The listing builds one solid part. Answer for the finished solid, in the listing's coordinates (mm). A direction names the side the tool comes from. Give positions to 0.01 mm unless a question says otherwise; leave off trailing zeros. Loops run counter-clockwise (first coordinate to the right, second up) from the corner with the lowest first, then second, coordinate; pieces in that order, holes last. Notation, with made-up numbers: (29, 8.5) - (83, 8.5) arc R26 ccw to (83, 36.5) - close; hole circle Ø5 at (-10, 30). An arc over 180 degrees is marked (long way). Write item = value, one per line. Start each with the question number.
1) Flat-ended cylindrical pins translate along their axes: P1, Ø5, axis at y = 4, z = -19.5, coming from the +X side; P2, Ø2, axis at x = -2, y = 5.5, coming from the -Z side; P3, Ø6, axis at y = -5, z = 2, coming from the -X side. Find the tip coordinate at first contact, or state that the pin passes through.
2) Which of the six approach directions +Z, -Z, +X, -X, +Y, -Y give full straight-line access (tool end or side, diameter ignored) to faces 1 (the flat face through (0, 0, 9.525)), 2 (the flat face through (-2, 3, 0))?
3) The part is cut by section D-D on z = 6. Write down the section's boundary in (x, y).
4) Consider probe 1 along Z at (x, y) = (-5.25, 2.5) (3 decimals); probe 2 along Z at (x, y) = (-1.5, 4.75) (3 decimals); probe 3 along Z at (x, y) = (3.5, 5) (3 decimals). Determine where each line is inside the solid, lowest interval first.
5) The part is cut by section C-C on z = -19. Write down the section's boundary in (x, y) (3 decimals), plus the area to 3 significant figures.
from build123d import *

# Parameters (mm, degrees)
SKETCH1_R           = 3.175
EXTRUDE1_DEPTH      = 25.4
CHAMFER2_SIZE       = 0.9525
SKETCH27_R          = 6.35
BOSS_EXTRUDE4_DEPTH = 3.175
SKETCH21_R          = 7.3421875
BOSS_EXTRUDE1_DEPTH = 6.35
CHAMFER3_SIZE       = 0.635


with BuildPart() as part:
    # Sketch1 → Extrude1 (new body)
    with BuildSketch(Plane.XY):
        Circle(SKETCH1_R)
    extrude(amount=-EXTRUDE1_DEPTH)

    # Chamfer2
    chamfer2_edges = [part.edges().sort_by_distance(p)[0] for p in [
        (-3.175, 0, -25.4),
    ]]
    chamfer(chamfer2_edges, length=CHAMFER2_SIZE)

    # Sketch27 → Boss-Extrude4 (add)
    with BuildSketch(Plane.XY):
        Circle(SKETCH27_R)
    extrude(amount=BOSS_EXTRUDE4_DEPTH)

    # Sketch21 → Boss-Extrude1 (add)
    with BuildSketch(Plane.XY.offset(3.175)):
        Circle(SKETCH21_R)
    extrude(amount=BOSS_EXTRUDE1_DEPTH)

    # Sketch28 → Cut-Revolve1 (revolve, cut)
    with BuildSketch(Plane(origin=(0, 0, 0), x_dir=(0, 0, -1), z_dir=(1, 0, 0))):
        with BuildLine():
            Line((-3.175, 6.35), (-0.635, 6.35))
            ThreePointArc((-0.635, 6.35), (-1.905, 5.469889405), (-3.175, 6.35))
        make_face()
    revolve(axis=Axis((0, 0, 0), (0, 0, -1)), mode=Mode.SUBTRACT)

    # Chamfer3
    chamfer3_edges = [part.edges().sort_by_distance(p)[0] for p in [
        (-7.3421875, 0, 3.175),
        (-7.3421875, 0, 9.525),
    ]]
    chamfer(chamfer3_edges, length=CHAMFER3_SIZE)


solid = part.part
Answer below:
q1.P1 = 2.8
q1.P2 = 0
q1.P3 = -6.86
q2.face_1 = +Z, +X, -X, +Y, -Y
q2.face_2 = -Z
q3.outline = circle Ø14.68 at (0, 0)
q4.probe_1 = 0 to 1.001, 2.809 to 9.525
q4.probe_2 = 0 to 9.525
q4.probe_3 = 0 to 0.757, 3.053 to 9.525
q5.outline = circle Ø6.35 at (0, 0)
q5.area = 31.7 mm2
